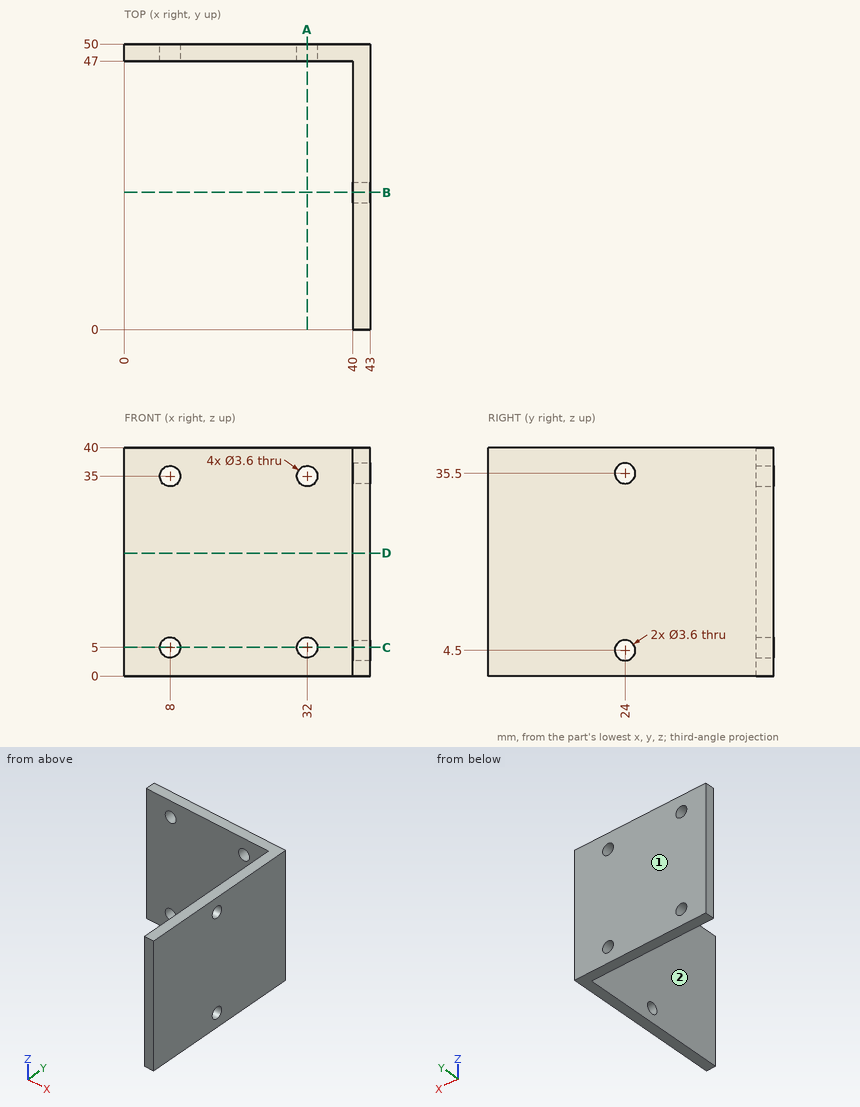
Geometry check sheet. Reference: drawing and pictorial views, mm from the part's lowest x, y, z. A direction names the side the tool comes from. Round coordinates to 2 decimals unless told otherwise and drop trailing zeros. Order: outer loops, then holes, each group sorted by start corner. A loop starts at its lowest first (then second) coordinate and runs counter-clockwise, first axis right, second up. Notation, with made-up numbers: (58, 26.25) - (110, 26.25) arc R19 cw to (110, 55.25) - close; hole circle Ø8 at (-9, -27). An arc over 180 degrees is marked (long way). Write item = value, one per line.
Q1. Section check A-A (x = 32). Record the boundary of the cut face in (y, z), and give its area (3 significant figures).
Computed:
outline = (47, 0) - (50, 0) - (50, 3.2) - (47, 3.2) - close; (47, 6.8) - (50, 6.8) - (50, 33.2) - (47, 33.2) - close; (47, 36.8) - (50, 36.8) - (50, 40) - (47, 40) - close
area = 98.4 mm^2
Q2. Go/stop test with flat-tipped pins: pin 1 (1 mm diameter, centred on x = 9, z = 24, fed in from -Y); pin 2 (8 mm diameter, centred on y = 10.5, z = 20.5, fed in from -X). Record where each tip stops, or that it passes through.
Computed:
pin_1 = 47
pin_2 = 40
Q3. Thickness scan on line 1 along Z through (x, y) = (8, 48.95); line 2 along X through (y, z) = (48.35, 35); line 3 along Y through (x, z) = (28, 13). Record the ranges inside material, lowest first.
Computed:
line_1 = 0 to 3.2, 6.8 to 33.2, 36.8 to 40
line_2 = 0 to 6.2, 9.8 to 30.2, 33.8 to 43
line_3 = 47 to 50
Q4. Tool access check on the marked faces 1 and 2. Record the directions out of +Z, -Z, +X, -X, +Y, -Y that give a thin tool (end or side, any length) a straight path to the whole face; none if there is none.
Computed:
face_1 = +Z, -Z, +X, -X, +Y
face_2 = +Z, -Z, -X, -Y
Q5. Section check B-B (y = 24). Record the boundary of the cut face in (x, z), and give its area (3 significant figures).
Computed:
outline = (40, 0) - (43, 0) - (43, 2.7) - (40, 2.7) - close; (40, 6.3) - (43, 6.3) - (43, 33.7) - (40, 33.7) - close; (40, 37.3) - (43, 37.3) - (43, 40) - (40, 40) - close
area = 98.4 mm^2
Q6. Section check D-D (z = 21.5). Record the boundary of the cut face in (x, y), and give its area (3 significant figures).
Computed:
outline = (0, 47) - (40, 47) - (40, 0) - (43, 0) - (43, 50) - (0, 50) - close
area = 270 mm^2
Q7. Section check C-C (z = 5). Record the boundary of the cut face in (x, y).
Computed:
outline = (0, 47) - (6.2, 47) - (6.2, 50) - (0, 50) - close; (9.8, 47) - (30.2, 47) - (30.2, 50) - (9.8, 50) - close; (33.8, 47) - (40, 47) - (40, 25.73) - (43, 25.73) - (43, 50) - (33.8, 50) - close; (40, 0) - (43, 0) - (43, 22.27) - (40, 22.27) - close
